```python
from build123d import *

# Parameters (mm, degrees)
BOSS_EXTRUDE1_DEPTH                  = 174.84725
F_10_32_TAPPED_HOLE1_D               = 4.0386
F_10_32_TAPPED_HOLE1_DEPTH           = 16.34744
F_10_32_TAPPED_HOLE1_TIP             = 1.213317848
F_10_32_TAPPED_HOLE1_ON_FACE_2_D     = 4.0386
F_10_32_TAPPED_HOLE1_ON_FACE_2_DEPTH = 16.34744
F_10_32_TAPPED_HOLE1_ON_FACE_2_TIP   = 1.213317848
SKETCH3_W                            = 0.889
SKETCH3_H                            = 1.0033


with BuildPart() as part:
    # Sketch1 → Boss-Extrude1 (new, symmetric)
    with BuildSketch(Plane.XY):
        with BuildLine():
            ThreePointArc((0.93173274, 6.79441227), (0, 6.858), (-0.93173274, 6.79441227))
            Line((-0.93173274, 6.79441227), (-5.41826726, 4.204110358))
            ThreePointArc((-5.41826726, 4.204110358), (-5.939202219, 3.429), (-6.35, 2.590301913))
            Line((-6.35, 2.590301913), (-6.35, -2.590301913))
            ThreePointArc((-6.35, -2.590301913), (-5.939202219, -3.429), (-5.41826726, -4.204110358))
            Line((-5.41826726, -4.204110358), (-0.93173274, -6.79441227))
            ThreePointArc((-0.93173274, -6.79441227), (0, -6.858), (0.93173274, -6.79441227))
            Line((0.93173274, -6.79441227), (5.41826726, -4.204110358))
            ThreePointArc((5.41826726, -4.204110358), (5.939202219, -3.429), (6.35, -2.590301913))
            Line((6.35, -2.590301913), (6.35, 2.590301913))
            ThreePointArc((6.35, 2.590301913), (5.939202219, 3.429), (5.41826726, 4.204110358))
            Line((5.41826726, 4.204110358), (0.93173274, 6.79441227))
        make_face()
    extrude(amount=BOSS_EXTRUDE1_DEPTH, both=True)

    # #10-32 Tapped Hole1
    with Locations(Plane.XY.offset(174.84725)):
        with Locations((0, 0)):
            Hole(F_10_32_TAPPED_HOLE1_D / 2, depth=F_10_32_TAPPED_HOLE1_DEPTH)
            with Locations((0, 0, -(F_10_32_TAPPED_HOLE1_DEPTH + F_10_32_TAPPED_HOLE1_TIP / 2))):  # 118° drill point
                Cone(0, F_10_32_TAPPED_HOLE1_D / 2, F_10_32_TAPPED_HOLE1_TIP, mode=Mode.SUBTRACT)

    # #10-32 Tapped Hole1 on face 2
    with Locations(Plane(origin=(0, 0, -174.84725), x_dir=(-1, 0, 0), z_dir=(0, 0, -1))):
        with Locations((0, 0)):
            Hole(F_10_32_TAPPED_HOLE1_ON_FACE_2_D / 2, depth=F_10_32_TAPPED_HOLE1_ON_FACE_2_DEPTH)
            with Locations((0, 0, -(F_10_32_TAPPED_HOLE1_ON_FACE_2_DEPTH + F_10_32_TAPPED_HOLE1_ON_FACE_2_TIP / 2))):  # 118° drill point
                Cone(0, F_10_32_TAPPED_HOLE1_ON_FACE_2_D / 2, F_10_32_TAPPED_HOLE1_ON_FACE_2_TIP, mode=Mode.SUBTRACT)

    # Sketch3 → Cut-Revolve1 (revolve, cut)
    with BuildSketch(Plane(origin=(0, 0, 0), x_dir=(0, 0, -1), z_dir=(1, 0, 0)), mode=Mode.PRIVATE) as cut_revolve1_sk:
        with Locations((-172.68825, 6.35635)):
            Rectangle(SKETCH3_W, SKETCH3_H)
    cut_revolve1 = revolve(cut_revolve1_sk.sketch.rotate(Axis((0, 0, 175.157387885), (0, 0, -1)), 90), axis=Axis((0, 0, 175.157387885), (0, 0, -1)), mode=Mode.SUBTRACT)

    # Mirror1: Cut-Revolve1 across plane
    add(cut_revolve1.mirror(Plane.XY), mode=Mode.SUBTRACT)


solid = part.part
```
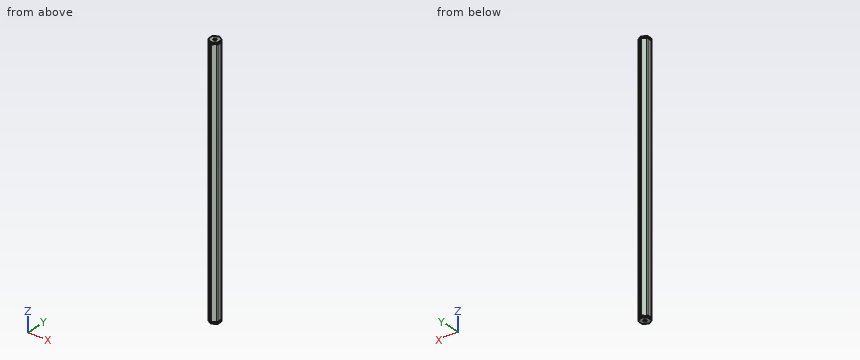
Geometry check sheet. Reference: the model listing, model coordinates, mm. Round coordinates to 2 decimals unless told otherwise and drop trailing zeros. Loops run counter-clockwise (first coordinate to the right, second up) from the corner with the lowest first, then second, coordinate; pieces in that order, holes last. Notation, with made-up numbers: (80.5, 69.25) -> (102.5, 69.25) arc R21 cw to (102.5, 96.25) -> close; hole circle Ø3 at (70.5, 83.25). An arc over 180 degrees is marked (long way). Use a Markdown table: item, result.
(1) Scan lines: probe 1 along X at (y, z) = (0, 166.75); probe 2 along Y at (x, z) = (2.5, 28); probe 3 along Y at (x, z) = (-0.5, 108.5). Record each from-to range of solid material in increasing order.
Calculated:
| item | result |
|---|---|
| probe 1 | -6.35 to -2.02, 2.02 to 6.35 |
| probe 2 | -5.89 to 5.89 |
| probe 3 | -6.84 to 6.84 |
(2) Sectioned sample at A-A (z = -52). Enter the section's corners in (x, y).
Calculated:
| item | result |
|---|---|
| outline | (-6.35, -2.59) arc R6.86 ccw to (-5.42, -4.2) -> (-0.93, -6.79) arc R6.86 ccw to (0.93, -6.79) -> (5.42, -4.2) arc R6.86 ccw to (6.35, -2.59) -> (6.35, 2.59) arc R6.86 ccw to (5.42, 4.2) -> (0.93, 6.79) arc R6.86 ccw to (-0.93, 6.79) -> (-5.42, 4.2) arc R6.86 ccw to (-6.35, 2.59) -> close |
(3) Go/stop test with a flat-tipped pin: P1, Ø2.5, axis at x = 0, y = 0, coming from the +Z side. Record where the tip stops, or that it passes through.
Calculated:
| item | result |
|---|---|
| P1 | z = 158.04 |
